Geometry: final body of the model. Coordinates: model frame, mm. Face numbers are marked on the shaded views. A direction names the side the tool comes from. Round coordinates to 2 decimals unless told otherwise and drop trailing zeros. Loops run counter-clockwise (first coordinate to the right, second up) from the corner with the lowest first, then second, coordinate; pieces in that order, holes last. Notation, with made-up numbers: (53.25, 9) - (99.25, 9) arc R10 ccw to (99.25, 14) - close; hole circle Ø10 at (31.5, -31.75). An arc over 180 degrees is marked (long way). Answer as CSV lines item,"result".
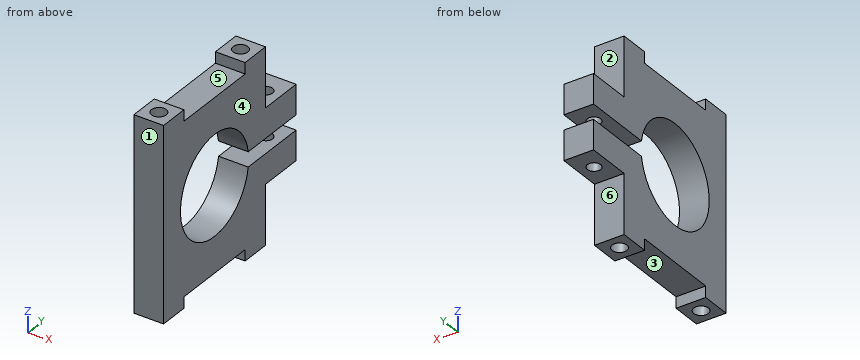
from build123d import *

# Parameters (mm, degrees)
CROQUIS1_W              = 65
CROQUIS1_H              = 50
CROQUIS1_R              = 16.7005
SALIENTE_EXTRUIR1_DEPTH = 5
CROQUIS2_W              = 7.5
CROQUIS2_H              = 30
CORTAR_EXTRUIR1_DEPTH   = 43.20485754
CROQUIS3_W              = 5
CROQUIS3_H              = 15
CORTAR_EXTRUIR2_DEPTH   = 43.20485754
CROQUIS4_W              = 10
CROQUIS4_H              = 15
SALIENTE_EXTRUIR2_DEPTH = 10
CROQUIS5_R              = 2.5
CORTAR_EXTRUIR3_DEPTH   = 10
CORTAR_EXTRUIR4_REACH   = 62.415
CROQUIS6_R              = 2.25


with BuildPart() as part:
    # Croquis1 → Saliente-Extruir1 (new, symmetric)
    with BuildSketch(Plane(origin=(0, 0, 0), x_dir=(0, 0, -1), z_dir=(1, 0, 0))):
        Rectangle(CROQUIS1_W, CROQUIS1_H)
        Circle(CROQUIS1_R, mode=Mode.SUBTRACT)
    extrude(amount=SALIENTE_EXTRUIR1_DEPTH, both=True)

    # Croquis2 → Cortar-Extruir1 (cut, through all)
    with BuildSketch(Plane(origin=(5, 0, 0), x_dir=(0, 0, -1), z_dir=(1, 0, 0))):
        with Locations((-32.5, 0)):
            Rectangle(CROQUIS2_W, CROQUIS2_H)
        with Locations((32.5, 0)):
            Rectangle(CROQUIS2_W, CROQUIS2_H)
    extrude(amount=-CORTAR_EXTRUIR1_DEPTH, mode=Mode.SUBTRACT)

    # Croquis3 → Cortar-Extruir2 (cut, through all)
    with BuildSketch(Plane(origin=(5, 0, 0), x_dir=(0, 0, -1), z_dir=(1, 0, 0))):
        with Locations((0, 20.85025)):
            Rectangle(CROQUIS3_W, CROQUIS3_H)
    extrude(amount=-CORTAR_EXTRUIR2_DEPTH, mode=Mode.SUBTRACT)

    # Croquis4 → Saliente-Extruir2 (add)
    with BuildSketch(Plane(origin=(5, 0, 0), x_dir=(0, 0, -1), z_dir=(1, 0, 0))):
        with Locations((-7.5, 32.5)):
            Rectangle(CROQUIS4_W, CROQUIS4_H)
        with Locations((7.5, 32.5)):
            Rectangle(CROQUIS4_W, CROQUIS4_H)
    extrude(amount=-SALIENTE_EXTRUIR2_DEPTH)

    # Croquis5 → Cortar-Extruir3 (cut)
    with BuildSketch(Plane.XY.offset(32.5)):
        with Locations((0, 20)):
            Circle(CROQUIS5_R)
        with Locations(Location((0, -20, 0), (0, 0, 180))):
            Circle(CROQUIS5_R)
    cortar_extruir3 = extrude(amount=-CORTAR_EXTRUIR3_DEPTH, mode=Mode.SUBTRACT)

    # Simetría1: Cortar-Extruir3 across plane
    add(cortar_extruir3.mirror(Plane.XY), mode=Mode.SUBTRACT)

    # Cortar-Extruir4: up to this face of the body (flat: up to its plane)
    cortar_extruir4_end = Plane(part.part.faces().sort_by_distance((0, 32.5, -12.5))[0])
    # Croquis6 → Cortar-Extruir4 (cut, up to the picked face)
    with BuildSketch(Plane.XY.offset(12.5), mode=Mode.PRIVATE) as cortar_extruir4_sk1:
        with Locations((0, 32.5)):
            Circle(CROQUIS6_R)
    cortar_extruir4_tool1 = split(extrude(cortar_extruir4_sk1.sketch, amount=-CORTAR_EXTRUIR4_REACH, mode=Mode.PRIVATE), bisect_by=cortar_extruir4_end, keep=Keep.BOTH, mode=Mode.PRIVATE)
    add(cortar_extruir4_tool1.solids().sort_by(Axis((0, 32.5, 12.5), (0, 0, -1)))[0], mode=Mode.SUBTRACT)


solid = part.part
(1) Material intervals for line 1 along Y through (x, z) = (0, -24.5); line 2 along Z through (x, y) = (-1, 36.5); line 3 along Y through (x, z) = (0, 4.5), sorted ascending.
Findings below:
line 1,"-25 to -22.5, -17.5 to 17.5, 22.5 to 25"
line 2,"-12.5 to -2.5, 2.5 to 12.5"
line 3,"-25 to -16.08, 16.08 to 30.25, 34.75 to 40"
(2) Section C-C (y = -20). Output: boundary loops of the cut face in (x, z), and give its area (3 significant figures).
Findings below:
outline,"(-5, -32.5) - (-2.5, -32.5) - (-2.5, -22.5) - (2.5, -22.5) - (2.5, -32.5) - (5, -32.5) - (5, 32.5) - (2.5, 32.5) - (2.5, 22.5) - (-2.5, 22.5) - (-2.5, 32.5) - (-5, 32.5) - close"
area,"550 mm2"
(3) Pin query (flat end, axial travel): P1, Ø4, axis at x = 0, y = -20, coming from the +Z side; P2, Ø1.5, axis at x = -2.5, y = 9.5, coming from the -Z side; P3, Ø4.5, axis at x = 0, y = -20, coming from the -Z side. Return the tip coordinate at first contact, or that it passes through.
Findings below:
P1,"z = 22.5"
P2,"z = -28.75"
P3,"z = -22.5"
(4) Section A-A (y = 32.5). Output: boundary loops of the cut face in (x, z).
Findings below:
outline,"(-5, -12.5) - (-2.25, -12.5) - (-2.25, -2.5) - (-5, -2.5) - close; (-5, 2.5) - (-2.25, 2.5) - (-2.25, 12.5) - (-5, 12.5) - close; (2.25, -12.5) - (5, -12.5) - (5, -2.5) - (2.25, -2.5) - close; (2.25, 2.5) - (5, 2.5) - (5, 12.5) - (2.25, 12.5) - close"
(5) Section D-D (x = 0). Give the number of separate pieces and of enclosed holes in the cut face, and give its area (3 significant figures).
Findings below:
separate pieces,"3"
enclosed holes,"0"
area,"2,120 mm2"
(6) Section B-B (x = 3.75). Output: boundary loops of the cut face in (y, z), and give its area (3 significant figures).
Findings below:
outline,"(-25, -32.5) - (-15, -32.5) - (-15, -28.75) - (15, -28.75) - (15, -32.5) - (25, -32.5) - (25, -12.5) - (40, -12.5) - (40, -2.5) - (16.51, -2.5) arc R16.7 cw (long way) to (16.51, 2.5) - (40, 2.5) - (40, 12.5) - (25, 12.5) - (25, 32.5) - (15, 32.5) - (15, 28.75) - (-15, 28.75) - (-15, 32.5) - (-25, 32.5) - close"
area,"2,410 mm2"
(7) Access query for the marked faces 1, 2 and 3. Directions: +Z, -Z, +X, -X, +Y, -Y. A direction counts if a zero-diameter tool reaches every point of the face in a straight line with its end or side. Return the directions, or none.
Findings below:
face 1,"+Z, -Z, +X, -X, -Y"
face 2,"+Z, +X, -X, +Y"
face 3,"-Z, +X, -X"
(8) Draft query along Y for the marked faces 4, 5 and 6. Return one class per face: pulls with the +Y half, pulls with the -Y half, needs draft (parallel to the pull), parting line crosses it, or undercut.
Findings below:
face 4,"needs draft"
face 5,"undercut"
face 6,"pulls with the +Y half"
